Verification items for the finished model (mm, model axes). A direction names the side the tool comes from. Coordinates: 2 decimals unless noted, no trailing zeros. Order: outer loops, then holes, each group sorted by start corner. A loop starts at its lowest first (then second) coordinate and runs counter-clockwise, first axis right, second up.
Q1. Cross-section at B-B, the plane z = -31. Record the boundary of the cut face in (x, y), and give its area (3 significant figures).
Q2. Draft check along X on faces 1 (the flat face through (-9, 10.312, 0)), 2 (the cylindrical face through (12.62, -29.66, 40.06)), 3 (the cylindrical face through (-12.57, -51.96, -0.43)). Enter one of: pulls with the +X half, pulls with the -X half, needs draft (parallel to the pull), parting line crosses it, or undercut.
Q3. Set-up check for faces 4 (the cylindrical face through (16.22, 29.44, -17.69)), 5 (the flat face through (-9, -31.688, 18)), 6 (the flat face through (-18, 38.312, 18)), 7 (the flat face through (15.4, -27.688, -37.1)): record each of +Z, -Z, +X, -X, +Y, -Y from which the full face is reachable in a straight line by a thin tool's end or side.
Q4. Cross-section at D-D, the plane x = -29. Record the boundary of the cut face in (y, z).
Q5. Thickness scan on line 1 (Y direction, x = -21, z = -2); line 2 (Y direction, x = -4, z = 19.5); line 3 (Z direction, x = 5.5, y = 26). Record the ranges inside material, lowest first.
Q6. Depth check by flat-ended pin: P1, Ø6, axis at x = 17, y = -1, coming from the -Z side; P2, Ø4, axis at x = -33, y = 16, coming from the -Z side; P3, Ø8, axis at x = -2.5, z = 32, coming from the -Y side; P4, Ø25, axis at x = -20.5, z = 8, coming from the -Y side. Enter the tip coordinate at first touch or a pass-through.
Q7. Cross-section at C-C, the plane y = -7. Record the boundary of the cut face in (x, z), and give its area (3 significant figures).
from build123d import *

# Parameters (mm, degrees)
SKETCH_1_R            = 21
EXTRUDE_1_DEPTH       = 17.5
SKETCH_2_W            = 1
SKETCH_2_H            = 31
SKETCH_3_R            = 12
CUT_EXTRUDE_1_DEPTH   = 9
SKETCH_4_R            = 9
EXTRUDE_2_DEPTH       = 16
HOLE_WIZARD_M4_2_D    = 3.3
HOLE_WIZARD_8_0_8_1_D = 8
CHAMFER_2_SIZE        = 0.5
SKETCH_15_R           = 10
CUT_EXTRUDE_3_DEPTH   = 5
SCALE1_SCALE          = 2


with BuildPart() as part:
    # 草图1 → 凸台-拉伸1 (new, symmetric)
    with BuildSketch(Plane(origin=(0, 0, 0), x_dir=(1, 0, 0), z_dir=(0, 1, 0))):
        with Locations(Location((0, 0, 0), (0, 0, 270))):
            Circle(SKETCH_1_R)
    extrude(amount=EXTRUDE_1_DEPTH, both=True)

    # 草图2 → 切除-旋转1 (revolve, cut)
    with BuildSketch(Plane.XY, mode=Mode.PRIVATE) as cut_revolve_1_sk:
        with Locations((20.5, 0)):
            Rectangle(SKETCH_2_W, SKETCH_2_H)
    revolve(cut_revolve_1_sk.sketch.rotate(Axis((0, 17.5, 0), (0, -1, 0)), 90), axis=Axis((0, 17.5, 0), (0, -1, 0)), mode=Mode.SUBTRACT)

    # 草图3 → 切除-拉伸1 (cut)
    with BuildSketch(Plane(origin=(0, 17.5, 0), x_dir=(1, 0, 0), z_dir=(0, 1, 0))):
        with Locations(Location((0, 0, 0), (0, 0, 270))):
            Circle(SKETCH_3_R)
    extrude(amount=-CUT_EXTRUDE_1_DEPTH, mode=Mode.SUBTRACT)

    # 草图4 → 凸台-拉伸2 (add)
    with BuildSketch(Plane.XZ.offset(17.5)):
        with Locations(Location((0, 0, 0), (0, 0, 90))):
            Circle(SKETCH_4_R)
    extrude(amount=EXTRUDE_2_DEPTH)

    # M4 螺纹孔2 (through all)
    with Locations(Plane(origin=(-43.616669336, 0, 0), x_dir=(0, 0, -1), z_dir=(-1, 0, 0))):
        with Locations((0, 26)):
            Hole(HOLE_WIZARD_M4_2_D / 2)

    # Ø8.0 (8) 直径孔1 (through all)
    with Locations(Plane(origin=(0, -33.5, 0), x_dir=(-1, 0, 0), z_dir=(0, -1, 0))):
        with Locations((0, 0)):
            Hole(HOLE_WIZARD_8_0_8_1_D / 2)

    # 倒角2
    chamfer_2_edges = [part.edges().sort_by_distance(p)[0] for p in [
        (0, -33.5, -9),
        (-4, -33.5, 0),
    ]]
    chamfer(chamfer_2_edges, length=CHAMFER_2_SIZE)

    # 草图15 → 切除-拉伸3 (cut)
    with BuildSketch(Plane(origin=(0, 8.5, 0), x_dir=(1, 0, 0), z_dir=(0, 1, 0))):
        with Locations(Location((0, 0, 0), (0, 0, 270))):
            Circle(SKETCH_15_R)
    extrude(amount=-CUT_EXTRUDE_3_DEPTH, mode=Mode.SUBTRACT)


with BuildPart() as part_1:
    # Scale1: scaled about (-1.22e-07, -3.311996838, 3.643e-06)
    add(part.part.scale(SCALE1_SCALE).moved(Location((1.22e-07, 3.311996838, -3.643e-06))))


solid = part_1.part
Check values:
1. outline: (-28.34, -31.69) - (28.34, -31.69) - (28.34, -27.69) - (25.28, -27.69) - (25.28, 34.31) - (28.34, 34.31) - (28.34, 38.31) - (-28.34, 38.31) - (-28.34, 34.31) - (-25.28, 34.31) - (-25.28, -27.69) - (-28.34, -27.69) - close
1. area: 3,590 mm2
2. face 1: undercut
2. face 2: parting line crosses it
2. face 3: needs draft
3. face 4: +Y
3. face 5: -Y
3. face 6: +Z, -Z, +X, -X, +Y
3. face 7: none
4. outline: (-31.69, -30.38) - (-27.69, -30.38) - (-27.69, -27.55) - (34.31, -27.55) - (34.31, -30.38) - (38.31, -30.38) - (38.31, 30.38) - (34.31, 30.38) - (34.31, 27.55) - (-27.69, 27.55) - (-27.69, 30.38) - (-31.69, 30.38) - close
5. line 1: y = -31.69 to 20.31
5. line 2: y = -31.69 to 10.31
5. line 3: z = -39.62 to -23.36, 23.36 to 39.62
6. P1: stops at z = -37.47
6. P2: stops at z = -25.28
6. P3: stops at y = -31.69
6. P4: stops at y = -63.69
7. outline: circle Ø80 at (0, 0); hole circle Ø16 at (0, 0)
7. area: 4,830 mm2
